from build123d import *

# Parameters (mm, degrees)
EXTRUDE_1_DEPTH                = 21
SKETCH_2_R                     = 13
EXTRUDE_2_DEPTH                = 123
CUT_EXTRUDE_START              = -17
CUT_EXTRUDE_1_DEPTH            = 17
CUT_EXTRUDE_2_DEPTH            = 17
SKETCH_5_R                     = 6
EXTRUDE_3_DEPTH                = 2
SKETCH_6_W                     = 2
SKETCH_6_H                     = 6
HOLE_WIZARD_M3_1_D             = 3.242
HOLE_WIZARD_M3_1_DEPTH         = 7
HOLE_WIZARD_M3_1_TIP           = 0.935884786
HOLE_WIZARD_M3_5_1_D           = 4.134
HOLE_WIZARD_M3_5_1_DEPTH       = 6
HOLE_WIZARD_M3_5_1_CBORE_D     = 8
HOLE_WIZARD_M3_5_1_CBORE_DEPTH = 0.5
HOLE_WIZARD_M3_5_2_D           = 4.134
HOLE_WIZARD_M3_5_2_DEPTH       = 6
HOLE_WIZARD_M3_5_2_CBORE_D     = 8
HOLE_WIZARD_M3_5_2_CBORE_DEPTH = 0.5
HOLE_WIZARD_M3_2_D             = 3.242
HOLE_WIZARD_M3_2_DEPTH         = 7
HOLE_WIZARD_M3_2_TIP           = 0.935884786
CHAMFER_1_SIZE                 = 0.433


with BuildPart() as part:
    # ｽｹｯﾁ1 → ﾎﾞｽ - 押し出し1 (new body)
    with BuildSketch(Plane(origin=(0, 0, 0), x_dir=(0, -1, 0), z_dir=(-1, 0, 0))):
        with BuildLine():
            Line((-5.499090807, -12.000000012), (5.499090807, -12.000000012))
            ThreePointArc((5.499090807, -12.000000012), (13.2, 0), (5.499090807, 12.000000012))
            Line((5.499090807, 12.000000012), (-5.499090807, 12.000000012))
            ThreePointArc((-5.499090807, 12.000000012), (-13.2, 0), (-5.499090807, -12.000000012))
        make_face()
    extrude(amount=-EXTRUDE_1_DEPTH)

    # ｽｹｯﾁ2 → ﾎﾞｽ - 押し出し2 (add)
    with BuildSketch(Plane(origin=(21, 0, 0), x_dir=(0, -1, 0), z_dir=(-1, 0, 0))):
        with Locations(Location((0, 0, 0), (0, 0, 112.619864808))):
            Circle(SKETCH_2_R)
    extrude(amount=-EXTRUDE_2_DEPTH)

    # ｽｹｯﾁ3 → ｶｯﾄ - 押し出し1 (cut)
    with BuildSketch(Plane(origin=(144, 0, 0), x_dir=(0, 0, -1), z_dir=(1, 0, 0)).offset(CUT_EXTRUDE_START)):
        with BuildLine():
            Line((-12, -5), (-12, 5))
            ThreePointArc((-12, 5), (-13, 0), (-12, -5))
        make_face()
    extrude(amount=CUT_EXTRUDE_1_DEPTH, mode=Mode.SUBTRACT)

    # ｽｹｯﾁ4 → ｶｯﾄ - 押し出し2 (cut)
    with BuildSketch(Plane(origin=(144, 0, 0), x_dir=(0, 0, -1), z_dir=(1, 0, 0)).offset(CUT_EXTRUDE_START)):
        with BuildLine():
            Line((12, 5), (12, -5))
            ThreePointArc((12, -5), (13, 0), (12, 5))
        make_face()
    extrude(amount=CUT_EXTRUDE_2_DEPTH, mode=Mode.SUBTRACT)

    # ｽｹｯﾁ5 → ﾎﾞｽ - 押し出し3 (add)
    with BuildSketch(Plane(origin=(144, 0, 0), x_dir=(0, 0, -1), z_dir=(1, 0, 0))):
        Circle(SKETCH_5_R)
    extrude(amount=EXTRUDE_3_DEPTH)

    # ｽｹｯﾁ6 → 回転1 (revolve)
    with BuildSketch(Plane.XY, mode=Mode.PRIVATE) as revolve_1_sk:
        with Locations((-1, 3)):
            Rectangle(SKETCH_6_W, SKETCH_6_H)
    revolve(revolve_1_sk.sketch.rotate(Axis((-2, 0, 0), (1, 0, 0)), 270), axis=Axis((-2, 0, 0), (1, 0, 0)))

    # ｽｹｯﾁ7 → ｶｯﾄ - 回転1 (revolve, cut)
    with BuildSketch(Plane.XY, mode=Mode.PRIVATE) as cut_revolve_1_sk:
        Polygon((-2, 4), (-2, 0), (99, 0), (99, 10), (19, 10), (19, 4), align=None)
    revolve(cut_revolve_1_sk.sketch.rotate(Axis((-2, 0, 0), (1, 0, 0)), 270), axis=Axis((-2, 0, 0), (1, 0, 0)), mode=Mode.SUBTRACT)

    # ｽｹｯﾁ8 → ｶｯﾄ - 回転2 (revolve, cut)
    with BuildSketch(Plane(origin=(16, 0, 0), x_dir=(0, 0, -1), z_dir=(1, 0, 0))):
        Polygon((-3.992522404, 12.702844697), (-5.578561032, 11.963262739), (-1.67721423, 3.596797524), (-1.224060337, 3.808106655), (-2.581245226, 6.718599042), (-1.674937439, 7.141217304), (-2.625828528, 9.180409824), (-2.504906146, 9.512641337), align=None)
    revolve(axis=Axis((16, 11.963262739, 5.578561032), (0, -0.9063077870366498, -0.42261826174069983)), mode=Mode.SUBTRACT)

    # ｽｹｯﾁ9 → ｶｯﾄ - 回転3 (revolve, cut)
    with BuildSketch(Plane(origin=(129, 0, 0), x_dir=(0, 0, -1), z_dir=(1, 0, 0))):
        Polygon((-3.907998745, 12.521583124), (-5.494037372, 11.782001166), (-0.921307811, 1.975750976), (-0.468153917, 2.187060107), (-2.581245226, 6.718599042), (-1.674937439, 7.141217304), (-2.625828528, 9.180409824), (-2.504906146, 9.512641337), align=None)
    revolve(axis=Axis((129, 11.782001166, 5.494037372), (0, -0.9063077870366498, -0.4226182617406999)), mode=Mode.SUBTRACT)

    # M3 すきま穴1
    with Locations(Plane(origin=(144, 0, 0), x_dir=(0, 0, -1), z_dir=(1, 0, 0))):
        with Locations((-7, 7), (-7, -7), (7, -7), (7, 7)):
            Hole(HOLE_WIZARD_M3_1_D / 2, depth=HOLE_WIZARD_M3_1_DEPTH)
            with Locations((0, 0, -(HOLE_WIZARD_M3_1_DEPTH + HOLE_WIZARD_M3_1_TIP / 2))):  # 120° drill point
                Cone(0, HOLE_WIZARD_M3_1_D / 2, HOLE_WIZARD_M3_1_TIP, mode=Mode.SUBTRACT)

    # M3.5 六角小ねじ用座ぐり穴1
    with Locations(Plane.XY.offset(12.000000012)):
        with Locations((11, 0), (133, 0)):
            CounterBoreHole(HOLE_WIZARD_M3_5_1_D / 2, HOLE_WIZARD_M3_5_1_CBORE_D / 2, HOLE_WIZARD_M3_5_1_CBORE_DEPTH, depth=HOLE_WIZARD_M3_5_1_DEPTH)

    # ｽｹｯﾁ14 → M3.5 皿頭小ねじ(100)用皿穴1 (revolve, cut)
    with BuildSketch(Plane(origin=(12, 12.999400949, -2.29214512), x_dir=(0, 0.17364817766692953, 0.9848077530122082), z_dir=(1, 0, 0))):
        Polygon((0, 0), (0, 6.193320669), (2.067, 4.999937663), (2.067, 0.432937663), (2.499937663, 0), align=None)
    revolve(axis=Axis((12, 19.252930181, -3.394811049), (0, -0.9848077530122082, 0.1736481776669295)), mode=Mode.SUBTRACT)

    # M3.5 六角小ねじ用座ぐり穴2
    with Locations(Plane(origin=(0, 0, -12.000000012), x_dir=(-1, 0, 0), z_dir=(0, 0, -1))):
        with Locations((-11, 0), (-133, 0)):
            CounterBoreHole(HOLE_WIZARD_M3_5_2_D / 2, HOLE_WIZARD_M3_5_2_CBORE_D / 2, HOLE_WIZARD_M3_5_2_CBORE_DEPTH, depth=HOLE_WIZARD_M3_5_2_DEPTH)

    # M3 すきま穴2
    with Locations(Plane.ZY):
        with Locations((7, 7), (7, -7), (-7, -7), (-7, 7)):
            Hole(HOLE_WIZARD_M3_2_D / 2, depth=HOLE_WIZARD_M3_2_DEPTH)
            with Locations((0, 0, -(HOLE_WIZARD_M3_2_DEPTH + HOLE_WIZARD_M3_2_TIP / 2))):  # 120° drill point
                Cone(0, HOLE_WIZARD_M3_2_D / 2, HOLE_WIZARD_M3_2_TIP, mode=Mode.SUBTRACT)

    # ｽｹｯﾁ20 → M3.5 皿頭小ねじ(100)用皿穴2 (revolve, cut)
    with BuildSketch(Plane(origin=(134, 12.802438431, -2.257415314), x_dir=(0, 0.1736481776669296, 0.9848077530122082), z_dir=(1, 0, 0))):
        Polygon((0, 0), (0, 6.193319686), (2.067, 4.99993668), (2.067, 0.43293668), (2.49993668, 0), align=None)
    revolve(axis=Axis((134, 19.055967663, -3.360081242), (0, -0.9848077530122082, 0.17364817766692964)), mode=Mode.SUBTRACT)

    # 面取り1
    chamfer_1_edges = [part.edges().sort_by_distance(p)[0] for p in [
        (13.067, 0, 11.500000012),
        (130.933, 0, -11.500000012),
        (8.933, 0, -11.500000012),
        (0, 7, -5.379),
        (0, -7, -5.379),
        (0, -7, 8.621),
        (0, 7, 8.621),
        (144, 7, -8.621),
        (144, -7, -8.621),
        (144, -7, 5.379),
        (144, 7, 5.379),
        (135.067, 0, 11.500000012),
    ]]
    chamfer(chamfer_1_edges, length=CHAMFER_1_SIZE)


solid = part.part
Input: part model. Units: mm. Frame: model coordinates. A direction names the side the tool comes from. Coordinates: 2 decimals unless noted, no trailing zeros. Write each loop counter-clockwise with the first axis right and the second up, starting at its lowest first coordinate (ties: lowest second). Pieces come first, ordered by that corner, then holes. Notation, with made-up numbers: M 78,70.5 L 113,70.5 A21 ccw 113,95.5 Z; hole C 12.25,-28.5 d3. An arc over 180 degrees is marked long. Answer as a JSON object with one key per item and string values. Group by question number.
(1) Section A-A on x = 31.5. Output: boundary loops of the cut face in (y, z).
(2) Set-up query: faces 1 (the face through (7.8, -2.4, 11.8)), 2 (the face through (11.7, 7.14, -1.06)), 3 (the face through (3.76, -5.9, -5.81)), 4 (the face through (8.935, 0.091, -8.498)), 5 (the face through (144, -0.3, 6.2)). Return all of +Z, -Z, +X, -X, +Y, -Y with unobstructed straight access to the full face (end or side cutting, diameter ignored); none if empty.
(3) Ray query, line 1 along Y through (x, z) = (76.5, 0); line 2 along Y through (x, z) = (140.25, -7); line 3 along Y through (x, z) = (3.75, -7). Return the intervals inside material, ascending. Write a range as [from, to].
(4) Section B-B on x = 125.5. Output: boundary loops of the cut face in (y, z), plus the area to 3 significant figures.
(5) Contact query for flat-ended pins moving along their axis: P1, Ø3.5, axis at x = 11, y = -2.5, coming from the -Z side; P2, Ø3, axis at x = 131, z = -9, coming from the -Y side; P3, Ø1.5, axis at x = 93, z = -3.5, coming from the +Y side. Output: stop coordinate, or through.
(6) Mould query, pull axis Z, two halves, no side actions, for faces 6 (the face through (137.3, -0.1, 12)), 7 (the face through (14.2, -2.4, -11.8)), 8 (the face through (17.476, 10.788, 3.993)). Classes: pulls with the +Z half, pulls with the -Z half, needs draft (parallel to the pull), parting line crosses it, or undercut.
Result set:
{
 "1": {"outline": "C 0,0 d26; hole C 0,0 d20"},
 "2": {"face 1": "+Z", "face 2": "none", "face 3": "-X", "face 4": "-Z", "face 5": "+X"},
 "3": {"line 1": "y = [-13, -10], [10, 13]", "line 2": "y = [-10.95, -8.62], [-5.38, 5.38], [8.62, 10.95]", "line 3": "y = [-11.19, -8.62], [-5.38, 5.38], [8.62, 11.19]"},
 "4": {"outline": "C 0,0 d26", "area": "531 mm2"},
 "5": {"P1": "stops at z = -12", "P2": "stops at y = -10.62", "P3": "stops at y = 12.71"},
 "6": {"face 6": "pulls with the +Z half", "face 7": "needs draft", "face 8": "undercut"}
}
